Check sheet for the modelled part. Datum: model origin and axes. Units: mm. Give positions to 0.01 mm unless a question says otherwise; leave off trailing zeros. Write each loop counter-clockwise with the first axis right and the second up, starting at its lowest first coordinate (ties: lowest second). Pieces come first, ordered by that corner, then holes. Notation, with made-up numbers: M 24.5,89.25 L 38.5,89.25 A28 cw 38.5,113.25 Z; hole C 14.25,85 d11. An arc over 180 degrees is marked long. One line per item, written item: value. Start each with the question number.
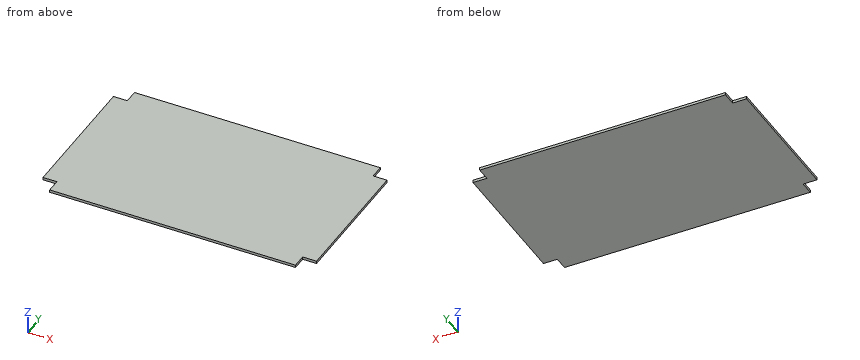
from build123d import *

# Parameters (mm, degrees)
SKETCH_1_W          = 500.8
SKETCH_1_H          = 300.8
EXTRUDE_1_DEPTH     = 4.75
SKETCH_2_W          = 25.4
SKETCH_2_H          = 25.4
CUT_EXTRUDE_1_DEPTH = 10


with BuildPart() as part:
    # 草圖1 → 填料-伸長1 (new body)
    with BuildSketch(Plane.XY):
        Rectangle(SKETCH_1_W, SKETCH_1_H)
    extrude(amount=EXTRUDE_1_DEPTH)

    # 草圖2 → 除料-伸長1 (cut)
    with BuildSketch(Plane(origin=(0, 0, 0), x_dir=(-1, 0, 0), z_dir=(0, 0, -1))):
        with Locations((-237.7, 137.7)):
            Rectangle(SKETCH_2_W, SKETCH_2_H)
        with Locations((-237.7, -137.7)):
            Rectangle(SKETCH_2_W, SKETCH_2_H)
        with Locations((237.7, 137.7)):
            Rectangle(SKETCH_2_W, SKETCH_2_H)
        with Locations((237.7, -137.7)):
            Rectangle(SKETCH_2_W, SKETCH_2_H)
    extrude(amount=-CUT_EXTRUDE_1_DEPTH, mode=Mode.SUBTRACT)


solid = part.part
1) Cross-section at A-A (z = 3.6). Record the boundary of the cut face in (x, y), plus the area to 3 significant figures.
2) Material ranges on L1, parallel to X at y = 131, z = 1.2, recorded low to high. Write a range as from..to.
3) Gauge pin test, flat ends, axial feed: pin 1 (1.5 mm diameter, centred on x = 9.5, y = -31, fed in from -Z); pin 2 (2.5 mm diameter, centred on x = -231.5, z = 1.5, fed in from -Y); pin 3 (1.4 mm diameter, centred on x = -241.5, z = 3.5, fed in from +Y); pin 4 (1.4 mm diameter, centred on y = -140, z = 2, fed in from +X). Record the tip position at first contact, or that the pin passes through.
Data:
1. outline: M -250.4,-125 L -225,-125 L -225,-150.4 L 225,-150.4 L 225,-125 L 250.4,-125 L 250.4,125 L 225,125 L 225,150.4 L -225,150.4 L -225,125 L -250.4,125 Z
1. area: 148,000 mm2
2. L1: x = -225..225
3. pin 1: stops at z = 0
3. pin 2: stops at y = -125
3. pin 3: stops at y = 125
3. pin 4: stops at x = 225
